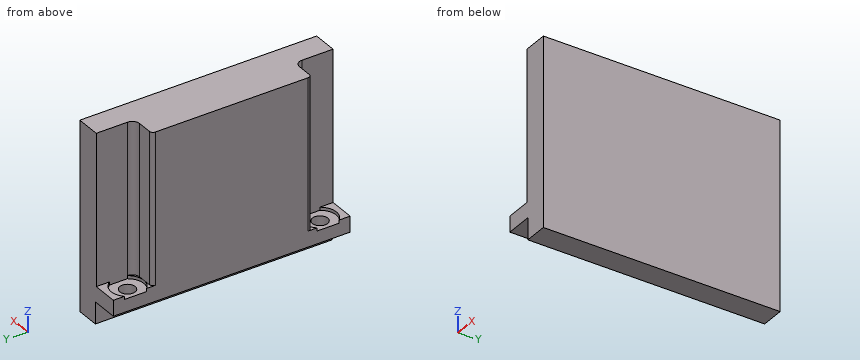
```python
from build123d import *

# Parameters (mm, degrees)
SKETCH_W        = 7.45
SKETCH_H        = 65.42
SKETCH_R        = 2.125
PAD_DEPTH       = 4.35
POCKET_DEPTH    = 0.85
POCKET_FACE1_W  = 65.42
POCKET_FACE1_H  = 4.35
PAD001_DEPTH    = 6.43
PAD001_FACE13_W = 65.42
PAD001_FACE13_H = 6.43
PAD002_DEPTH    = 6
PAD003_DEPTH    = 41.65
FILLET_R        = 2
FILLET001_R     = 1


with BuildPart() as part:
    # Sketch → Pad (new body)
    with BuildSketch(Plane.XY):
        Rectangle(SKETCH_W, SKETCH_H)
        with Locations((-0.43, -26.585)):
            Circle(SKETCH_R, mode=Mode.SUBTRACT)
        with Locations((-0.43, 26.585)):
            Circle(SKETCH_R, mode=Mode.SUBTRACT)
    extrude(amount=PAD_DEPTH)

    # Sketch001 (on DatumPlane) → Pocket (cut)
    with BuildSketch(Plane.XY.offset(4.35)):
        with BuildLine():
            ThreePointArc((3.345, -24.135638), (-0.039757, -22.101953), (-3.725, -23.520204))
            Line((-3.725, -23.520204), (-3.725, -29.649796))
            ThreePointArc((-3.725, -29.649796), (-0.039757, -31.068047), (3.345, -29.034362))
            Line((3.345, -24.135638), (3.345, -29.034362))
        make_face()
        with BuildLine():
            ThreePointArc((-3.725, 23.520204), (-0.039757, 22.101953), (3.345, 24.135638))
            Line((3.345, 29.034362), (3.345, 24.135638))
            ThreePointArc((3.345, 29.034362), (-0.039757, 31.068047), (-3.725, 29.649796))
            Line((-3.725, 29.649796), (-3.725, 23.520204))
        make_face()
    extrude(amount=-POCKET_DEPTH, mode=Mode.SUBTRACT)

    # Pocket Face1 → Pad001 (add)
    with BuildSketch(Plane(origin=(3.725, 0, 2.175), x_dir=(0, -1, 0), z_dir=(1, 0, 0))):
        Rectangle(POCKET_FACE1_W, POCKET_FACE1_H)
    extrude(amount=PAD001_DEPTH)

    # Pad001 Face13 → Pad002 (add)
    with BuildSketch(Plane(origin=(6.94, 0, 0), x_dir=(0, -1, 0), z_dir=(0, 0, -1))):
        Rectangle(PAD001_FACE13_W, PAD001_FACE13_H)
    extrude(amount=PAD002_DEPTH)

    # Sketch002 (on Face5 of Pad002) → Pad003 (join)
    with BuildSketch(Plane.XY.offset(4.35)):
        Polygon((10.155, 32.71), (10.155, -32.71), (3.345, -32.71), (3.345, -22.085), (-3.725, -22.085), (-3.725, 22.085), (3.345, 22.085), (3.345, 32.71), align=None)
    extrude(amount=PAD003_DEPTH)

    # Fillet
    fillet_edges = [part.edges().sort_by_distance(p)[0] for p in [
        (3.345, -22.085, 25.175),
        (3.345, 22.085, 25.175),
    ]]
    fillet(fillet_edges, radius=FILLET_R)

    # Fillet001
    fillet001_edges = [part.edges().sort_by_distance(p)[0] for p in [
        (-3.725, -22.085, 25.175),
        (-3.725, 22.085, 25.175),
    ]]
    fillet(fillet001_edges, radius=FILLET001_R)


solid = part.part
```
The model under review builds one solid part; all positions refer to its coordinate system, in mm. Round coordinates to 2 decimals unless told otherwise and drop trailing zeros. Order: outer loops, then holes, each group sorted by start corner. A loop starts at its lowest first (then second) coordinate and runs counter-clockwise, first axis right, second up. Notation, with made-up numbers: M -21.5,49.25 L 22.5,49.25 A9 cw 22.5,56.25 Z; hole C 55.25,-1 d4. An arc over 180 degrees is marked long. Use a Markdown table: item, result.
1) Wall thickness on line 1 along Y through (x, z) = (-0.43, 2.05); line 2 along Y through (x, z) = (-0.25, 31) (3 decimals); line 3 along X through (y, z) = (-27.5, -0.5) (3 decimals): over which ranges is each line inside the solid? List them lowest first. Write a range as [from, to].
Report:
| item | result |
|---|---|
| line 1 | [-32.71, -28.71], [-24.46, 24.46], [28.71, 32.71] |
| line 2 | [-22.085, 22.085] |
| line 3 | [3.725, 10.155] |
2) Insertion check: pin 1 (1.2 mm diameter, centred on x = -1, z = 23.5, fed in from -Y) (3 decimals); pin 2 (2 mm diameter, centred on x = 1, y = -27.5, fed in from +Z); pin 3 (4 mm diameter, centred on x = 1, y = -30.5, fed in from +Z). Each pin has a flat end and moves straight along its axis. Give the tip position at first contact, or say it passes through.
Report:
| item | result |
|---|---|
| pin 1 | y = -22.085 |
| pin 2 | z = 3.5 |
| pin 3 | z = 4.35 |
3) Consider section A-A (z = 18.5). Write out the cut boundary in (x, y) (3 decimals).
Report:
| item | result |
|---|---|
| outline | M -3.725,-21.085 A1 ccw -2.725,-22.085 L 1.345,-22.085 A2 cw 3.345,-24.085 L 3.345,-32.71 L 10.155,-32.71 L 10.155,32.71 L 3.345,32.71 L 3.345,24.085 A2 cw 1.345,22.085 L -2.725,22.085 A1 ccw -3.725,21.085 Z |
4) Consider section B-B (y = 5.5). Write out the cut boundary in (x, z) (3 decimals).
Report:
| item | result |
|---|---|
| outline | M -3.725,0 L 3.725,0 L 3.725,-6 L 10.155,-6 L 10.155,46 L -3.725,46 Z |
5) Consider section C-C (z = 1.5). Write out the cut boundary in (x, y) (3 decimals), then the cut area to 3 significant figures.
Report:
| item | result |
|---|---|
| outline | M -3.725,-32.71 L 10.155,-32.71 L 10.155,32.71 L -3.725,32.71 Z; hole C -0.43,-26.585 d4.25; hole C -0.43,26.585 d4.25 |
| area | 880 mm^2 |
